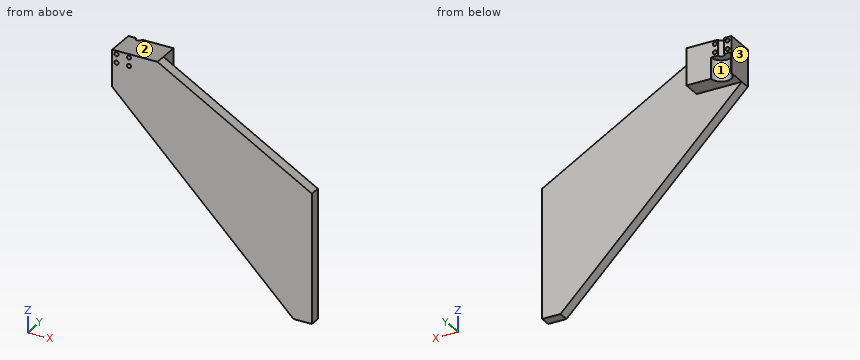
Autodesk Inventor part; units mm, degrees
ref_plane "YZ Plane" through (0, 0, 0) normal (1, 0, 0) x (0, 1, 0)
ref_plane "XZ Plane" through (0, 0, 0) normal (0, 1, 0) x (-1, 0, 0)
ref_plane "XY Plane" through (0, 0, 0) normal (0, 0, 1) x (1, 0, 0)
sketch "Sketch1" plane through (0, 0, 0) normal (0, 1, 0) x (-1, 0, 0)
  line L0 (111.9461, 87.1683) -> (-118.0539, 87.1683)
  line L1 (-118.0539, 87.1683) -> (-118.0539, -87.8317)
  line L2 (-118.0539, -87.8317) -> (111.9461, -87.8317)
  line L3 (111.9461, -87.8317) -> (111.9461, 87.1683)
  line L4 (111.9461, 52.1683) -> (-28.0539, -87.8317)
  point P0 (0, 0)
  dimension "d0" = 175
  dimension "d1" = 230
  dimension "d2" = 45
  dimension "d3" = 35
extrude "Extrusion1" add sketch "Sketch1" along normal blind 10 contours L3 L4 L2 L1 L0
sketch "Sketch2" plane through (0, 10, 0) normal (0, 1, 0) x (1, 0, 0)
  line L0 (-111.9461, -52.1683) -> (-111.9461, -87.1683)
  line L1 (-111.9461, -87.1683) -> (-69, -87.1683)
  line L2 (-69, -87.1683) -> (-69, -52.1683)
  line L3 (-69, -52.1683) -> (-111.9461, -52.1683)
  line L4 (-111.9461, -52.1683) -> (-111.9461, -87.1683)
  point P0 (0, 0)
extrude "Extrusion2" add sketch "Sketch2" along normal blind 17
sketch "Sketch3" plane through (-111.9461, 0, 87.1683) normal (0, 0, 1) x (1, 0, 0)
  line L0 (0, 27) -> (42.9461, 27)
  circle A0 centre (10, 27) radius 2.9
  point P0 (111.9461, 0)
  point P1 (12.9, 27)
  point P2 (7.1, 27)
  dimension "d12" = 5.8
extrude "Extrusion3" cut sketch "Sketch3" against normal blind 40 contours L0 A0 picked at (10.9386, 26.7687)
sketch "Sketch4" plane through (-69, 10, 52.1683) normal (0, 0, -1) x (-1, 0, 0)
  arc A0 (30.0461, 17) -> (35.8461, 17) centre (32.9461, 17) ccw
  circle A1 centre (32.9461, 17) radius 9.6071
  point P0 (-69, -10)
extrude "Extrusion4" cut sketch "Sketch4" against normal blind 20
sketch "Sketch5" plane through (0, 27, 0) normal (0, 1, 0) x (1, 0, 0)
  circle A0 centre (-108, -84) radius 2
  circle A1 centre (-108, -76) radius 2
  circle A2 centre (-96, -76) radius 2
  circle A3 centre (-96, -84) radius 2
  point P0 (0, 0)
extrude "Extrusion5" cut sketch "Sketch5" against normal blind 40
sketch "Sketch6" plane through (0, 10, 0) normal (0, 1, 0) x (1, 0, 0)
  line L0 (-111.9461, -87.1683) -> (118.0539, -87.1683)
  line L1 (118.0539, -87.1683) -> (118.0539, 87.8317)
  line L2 (-99.0461, -87.1683) -> (-69, -87.1683)
  line L3 (-69, -87.1683) -> (118.0539, 20.8273)
  point P0 (0, 0)
  dimension "d18" = 30
extrude "Extrusion6" cut sketch "Sketch6" against normal blind 40
sketch "Sketch7" plane through (0, 10, 0) normal (0, 1, 0) x (1, 0, 0)
  line L0 (28.0539, 87.8317) -> (-111.9461, -52.1683)
  line L1 (28.0539, 87.8317) -> (93.621, 153.3988)
  line L2 (93.621, 153.3988) -> (118.0539, 153.3988)
  line L3 (118.0539, 20.8273) -> (118.0539, 87.8317)
  line L4 (118.0539, 153.3988) -> (118.0539, 87.8317)
  line L5 (28.0539, 87.8317) -> (118.0539, 87.8317)
  point P0 (0, 0)
extrude "Extrusion7" add sketch "Sketch7" against normal blind 10
sketch "Sketch8" plane through (0, 10, 0) normal (0, 1, 0) x (1, 0, 0)
  line L0 (118.0539, 20.8273) -> (118.0539, 153.3988)
  line L1 (118.0539, 153.3988) -> (77.5539, 153.3988)
  line L2 (77.5539, 153.3988) -> (77.5539, -53)
  line L3 (77.5539, -53) -> (118.0539, -53)
  line L4 (118.0539, -53) -> (118.0539, 153.3988)
  line L5 (77.5539, 153.3988) -> (12, 153.3988)
  line L6 (12, 153.3988) -> (12, 120)
  line L7 (12, 120) -> (77.5539, 120)
  line L8 (77.5539, 120) -> (77.5539, 153.3988)
  point P0 (0, 0)
  dimension "d23" = 40.5
extrude "Extrusion8" cut sketch "Sketch8" against normal blind 10
properties part number "Z_babka"
Read the model definition and answer for the solid it produces. Units are mm, in the model's axes. Face numbers are marked on the shaded views. Coordinates: 2 decimals unless noted, no trailing zeros. Write each loop counter-clockwise with the first axis right and the second up, starting at its lowest first coordinate (ties: lowest second). Pieces come first, ordered by that corner, then holes. Notation, with made-up numbers: (-23, 51.25) - (18, 51.25) arc R22 cw to (18, 59.25) - close; hole circle Ø5 at (-34.5, -5.5). An arc over 180 degrees is marked (long way). One line per question, with ' | ' between items.
Q1. Find section A-A, the plane y = 3. Write down the section's boundary in (x, z), plus the area to 3 significant figures.
Result set:
outline: (-111.95, 52.17) - (60.22, -120) - (77.55, -120) - (77.55, 2.56) - (-69, 87.17) - (-111.95, 87.17) - close; hole circle Ø4 at (-108, 76); hole circle Ø4 at (-108, 84); hole circle Ø4 at (-96, 76); hole circle Ø4 at (-96, 84) | area: 18,200 mm^2
Q2. Find section D-D, the plane y = 21.5. Write down the section's boundary in (x, z).
Result set:
outline: (-111.95, 52.17) - (-109.82, 52.17) - (-109.82, 72.17) - (-94.07, 72.17) - (-94.07, 52.17) - (-69, 52.17) - (-69, 87.17) - (-111.95, 87.17) - close; hole circle Ø4 at (-108, 76); hole circle Ø4 at (-108, 84); hole circle Ø4 at (-96, 76); hole circle Ø4 at (-96, 84)
Q3. Consider L1, parallel to X at y = 12.75, z = 76; L2, parallel to Z at x = -108, y = 19.75; L3, parallel to X at y = 7.25, z = 84. Determine where each line is inside the solid, lowest interval first. Write a range as [from, to].
Result set:
L1: [-111.95, -110], [-106, -98], [-94, -69] | L2: [72.17, 74], [78, 82], [86, 87.17] | L3: [-111.95, -110], [-106, -98], [-94, -63.51]
Q4. Find section C-C, the plane x = 2. Write down the section's boundary in (y, z).
Result set:
outline: (0, -61.78) - (10, -61.78) - (10, 46.18) - (0, 46.18) - close
Q5. Each of these flat-tipped pins is pushed along its axis until it touches: P1, Ø5, axis at x = -96, z = 76, coming from the -Y side; P2, Ø10.5, axis at x = -101, y = 20, coming from the -Z side; P3, Ø12, axis at y = 19, z = -55, coming from the -X side; P4, Ø4, axis at x = 48.5, z = -31.5, coming from the +Y side. Where does it stop, or does it pass through?
Result set:
P1: y = 0 | P2: z = 52.17 | P3: through | P4: y = 10
Q6. Determine the mould class of the marked faces 1, 2 and 3 for opening direction X: +X half, -X half, draft (parallel to the pull), parting line (faces both ways), or undercut.
Result set:
face 1: undercut | face 2: draft | face 3: -X half
Q7. Find section B-B, the plane z = 66. Write down the section's boundary in (x, y), plus the area to 3 significant figures.
Result set:
outline: (-111.95, 0) - (-32.34, 0) - (-32.34, 10) - (-69, 10) - (-69, 27) - (-92.34, 27) arc R9.61 cw to (-111.55, 27) - (-111.95, 27) - close | area: 1,380 mm^2
